Check sheet for the drawn part. Datum: minimum x, y, z corner. Units: mm. A direction names the side the tool comes from. Coordinates: 2 decimals unless noted, no trailing zeros. Write each loop counter-clockwise with the first axis right and the second up, starting at its lowest first coordinate (ties: lowest second). Pieces come first, ordered by that corner, then holes. Notation, with made-up numbers: (52, 8.25) -> (81, 8.25) arc R15 cw to (81, 23.25) -> close; hole circle Ø2 at (-35, 58.25). An arc over 180 degrees is marked (long way). One line per question, with ' | ' between items.
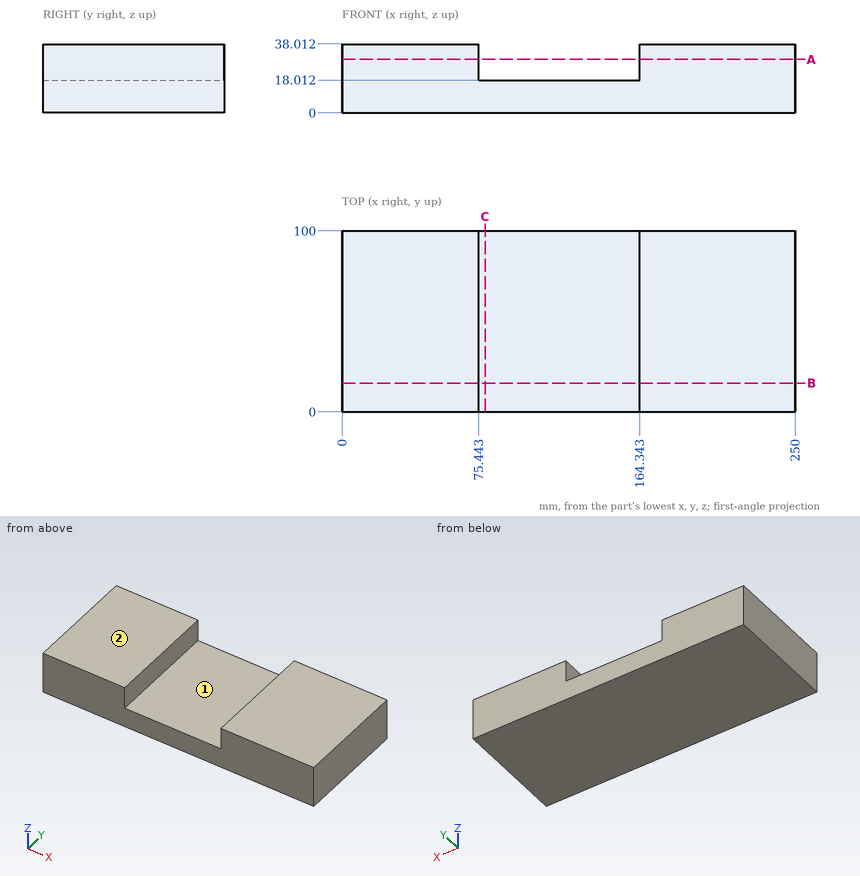
1. Material ranges on line 1 (X direction, y = 72.5, z = 25); line 2 (Z direction, x = 161.5, y = 86), recorded low to high. Write a range as from..to.
Worked answers:
line 1: 0..75.44, 164.34..250 | line 2: 0..18.01
2. Cross-section at B-B on y = 16. Record the boundary of the cut face in (x, z).
Worked answers:
outline: (0, 0) -> (250, 0) -> (250, 38.01) -> (164.34, 38.01) -> (164.34, 18.01) -> (75.44, 18.01) -> (75.44, 38.01) -> (0, 38.01) -> close
3. Cross-section at C-C on x = 79. Record the boundary of the cut face in (y, z).
Worked answers:
outline: (0, 0) -> (100, 0) -> (100, 18.01) -> (0, 18.01) -> close
4. Tool access check on the marked faces 1 and 2. Record the directions out of +Z, -Z, +X, -X, +Y, -Y that give a thin tool (end or side, any length) a straight path to the whole face; none if there is none.
Worked answers:
face 1: +Z, +Y, -Y | face 2: +Z, +X, -X, +Y, -Y
5. Cross-section at A-A on z = 29.5. Record the boundary of the cut face in (x, y).
Worked answers:
outline: (0, 0) -> (75.44, 0) -> (75.44, 100) -> (0, 100) -> close; (164.34, 0) -> (250, 0) -> (250, 100) -> (164.34, 100) -> close
